Build history of the part. All positions in model axes, mm. A direction names the side the tool comes from. Give positions to 0.01 mm unless a question says otherwise; leave off trailing zeros. Loops run counter-clockwise (first coordinate to the right, second up) from the corner with the lowest first, then second, coordinate; pieces in that order, holes last. Notation, with made-up numbers: (-20.5, 31) -> (23.5, 31) arc R14 cw to (23.5, 49) -> close; hole circle Ø6 at (50, 83.5). An arc over 180 degrees is marked (long way). One line per question, with ' | ' between items. Start each with the question number.
(1) Drill centre lines: L1, parallel to Z at x = -6, y = -7.25; L2, parallel to Y at x = 6, z = 99; L3, parallel to Z at x = -3.5, y = -1.25. Where is each one in solid material? Low to high. Write a range as from..to.
(2) Flat gauge pins, fed straight in: pin 1 Ø2 at (y, z) = (-7, 84.5) entering from -X; pin 2 Ø8.5 at (y, z) = (1, 4.5) entering from +X; pin 3 Ø5 at (x, y) = (2.5, 7) entering from -Z; pin 4 Ø6 at (x, z) = (-8, 72) entering from +Y. Where does each tip first touch, or does it go through?
(3) Slice it at D-D, the plane z = 35.5. Write the cut outline in (x, y), then the cut area to 3 significant figures.
(4) Slice it at B-B, the plane x = -4.5. Write the cut outline in (y, z), then the cut area to 3 significant figures.
(5) 3-axis set-ups, long thin cutter, end or side, ignore diameter. For faces 1 (the face through (7, 0, 15)), 2 (the face through (6, -0.1, 5.7)), 3 (the face through (0, 0, 20)), 4 (the face through (-4.5, -7.4, 26)), 5 (the face through (0, 3, 144)): which of +Z, -Z, +X, -X, +Y, -Y reach the whole face in a straight line?
(6) Slice it at C-C, the plane z = 145.5. Write the cut outline in (x, y).
(7) Mould opens along X. For faces 6 (the face through (0, -5, 18)), 7 (the face through (-6, 0.1, 5.7)), 8 (the face through (-1.73, -7.81, 148.9)) say: pulls with the +X half, pulls with the -X half, needs draft (parallel to the pull), parting line crosses it, or undercut.
(8) Slice it at A-A, the plane z = 9. Write the cut outline in (x, y).
```python
from build123d import *

# Parameters (mm, degrees)
EXTRUDE_1_DEPTH     = 15
SKETCH_2_R          = 3
CUT_EXTRUDE_1_DEPTH = 21.808652047
SKETCH_3_R          = 10
EXTRUDE_2_DEPTH     = 11
SKETCH_4_R          = 2.5
CUT_EXTRUDE_3_DEPTH = 10
SKETCH_5_R          = 8.5
SKETCH_5_R_2        = 8
EXTRUDE_4_DEPTH     = 105
SKETCH_6_R          = 10
EXTRUDE_5_DEPTH     = 11
SKETCH_7_R          = 2.5
CUT_EXTRUDE_4_DEPTH = 10
SKETCH_8_R          = 8
EXTRUDE_6_DEPTH     = 14
SKETCH_9_R          = 3
CUT_EXTRUDE_5_DEPTH = 100


with BuildPart() as part:
    # 草图1 → 凸台-拉伸1 (new body)
    with BuildSketch(Plane.XY):
        with BuildLine():
            ThreePointArc((0, 8), (-3.291502622, 7.291502622), (-6, 5.291502622))
            Line((-6, 5.291502622), (-6, -5.291502622))
            ThreePointArc((-6, -5.291502622), (-3.291502622, -7.291502622), (0, -8))
            Line((0, -8), (0, 8))
        make_face()
        with BuildLine():
            ThreePointArc((6, 5.291502622), (3.291502622, 7.291502622), (0, 8))
            Line((0, 8), (0, -8))
            ThreePointArc((0, -8), (3.291502622, -7.291502622), (6, -5.291502622))
            Line((6, -5.291502622), (6, 5.291502622))
        make_face()
    extrude(amount=EXTRUDE_1_DEPTH)

    # 草图2 → 切除-拉伸1 (cut, through all)
    with BuildSketch(Plane.ZY.offset(6)):
        with Locations((9, 0)):
            Circle(SKETCH_2_R)
    extrude(amount=-CUT_EXTRUDE_1_DEPTH, mode=Mode.SUBTRACT)

    # 草图3 → 凸台-拉伸2 (add)
    with BuildSketch(Plane.XY.offset(15)):
        Circle(SKETCH_3_R)
    extrude(amount=EXTRUDE_2_DEPTH)

    # 草图4 → 切除-拉伸3 (cut)
    with BuildSketch(Plane(origin=(0, 0, 0), x_dir=(1, 0, 0), z_dir=(0, 1, 0))):
        with Locations(Location((0, -20.5, 0), (0, 0, 270))):
            Circle(SKETCH_4_R)
    extrude(amount=-CUT_EXTRUDE_3_DEPTH, mode=Mode.SUBTRACT)

    # 草图5 → 凸台-拉伸4 (add)
    with BuildSketch(Plane.XY.offset(26)):
        Circle(SKETCH_5_R)
        Circle(SKETCH_5_R_2, mode=Mode.SUBTRACT)
    extrude(amount=EXTRUDE_4_DEPTH)

    # 草图6 → 凸台-拉伸5 (add)
    with BuildSketch(Plane.XY.offset(131)):
        Circle(SKETCH_6_R)
    extrude(amount=EXTRUDE_5_DEPTH)

    # 草图7 → 切除-拉伸4 (cut)
    with BuildSketch(Plane(origin=(0, 0, 0), x_dir=(1, 0, 0), z_dir=(0, 1, 0))):
        with Locations(Location((0, -136.5, 0), (0, 0, 270))):
            Circle(SKETCH_7_R)
    extrude(amount=-CUT_EXTRUDE_4_DEPTH, mode=Mode.SUBTRACT)

    # 草图8 → 凸台-拉伸6 (add)
    with BuildSketch(Plane.XY.offset(142)):
        Circle(SKETCH_8_R)
    extrude(amount=EXTRUDE_6_DEPTH)

    # 草图9 → 切除-拉伸5 (cut)
    with BuildSketch(Plane.XY.offset(156)):
        Circle(SKETCH_9_R)
    extrude(amount=-CUT_EXTRUDE_5_DEPTH, mode=Mode.SUBTRACT)


solid = part.part
```
Final values:
1) L1: 15..26, 131..142 | L2: -6.02..-5.29, 5.29..6.02 | L3: 0..6.27, 11.73..26, 131..156
2) pin 1: x = -6.02 | pin 2: x = 6 | pin 3: z = 0 | pin 4: y = 6.87
3) outline: circle Ø17 at (0, 0); hole circle Ø16 at (0, 0) | area: 25.9 mm2
4) outline: (-8.93, 15) -> (-6.61, 15) -> (-6.61, 0) -> (6.61, 0) -> (6.61, 15) -> (8.93, 15) -> (8.93, 26) -> (7.21, 26) -> (7.21, 131) -> (8.93, 131) -> (8.93, 142) -> (6.61, 142) -> (6.61, 156) -> (-6.61, 156) -> (-6.61, 142) -> (-8.93, 142) -> (-8.93, 131) -> (-7.21, 131) -> (-7.21, 26) -> (-8.93, 26) -> close; hole (-6.61, 26) -> (6.61, 26) -> (6.61, 131) -> (-6.61, 131) -> close; hole circle Ø6 at (0, 9) | area: 874 mm2
5) face 1: -Z | face 2: -Z, +X, +Y, -Y | face 3: -Y | face 4: none | face 5: +Z
6) outline: circle Ø16 at (0, 0); hole circle Ø6 at (0, 0)
7) face 6: undercut | face 7: pulls with the -X half | face 8: parting line crosses it
8) outline: (-6, -5.29) arc R8 ccw to (6, -5.29) -> (6, -3) -> (-6, -3) -> close; (-6, 3) -> (6, 3) -> (6, 5.29) arc R8 ccw to (-6, 5.29) -> close
